CAD build for the part. Positions are in the model's coordinates, mm. A direction names the side the tool comes from. Coordinates: 2 decimals unless noted, no trailing zeros. Loops run counter-clockwise (first coordinate to the right, second up) from the corner with the lowest first, then second, coordinate; pieces in that order, holes last. Notation, with made-up numbers: (57, -10) -> (79, -10) arc R20 cw to (79, 19) -> close; hole circle Ø11 at (-31, 16). An arc over 180 degrees is marked (long way). Answer as CSV lines item,"result". Start each with the question number.
Autodesk Inventor part; units mm, degrees
ref_plane "YZ Plane" through (0, 0, 0) normal (1, 0, 0) x (0, 1, 0)
ref_plane "XZ Plane" through (0, 0, 0) normal (0, 1, 0) x (-1, 0, 0)
ref_plane "XY Plane" through (0, 0, 0) normal (0, 0, 1) x (1, 0, 0)
sketch "Sketch1" plane through (0, 0, 0) normal (0, 1, 0) x (-1, 0, 0)
  line L0 (-7.5, 35) -> (7.5, 35)
  line L1 (7.5, 35) -> (7.5, -35)
  line L2 (7.5, -35) -> (-7.5, -35)
  line L3 (-7.5, -35) -> (-7.5, 35)
  line L4 (-7.5, 35) -> (7.5, -35) construction
  line L5 (7.5, 35) -> (-7.5, -35) construction
  circle A0 centre (0, 17) radius 1.75
  circle A1 centre (0, -17) radius 1.75
  point P0 (0, 0)
  point P1 (0, -35)
  dimension "d0" = 15
  dimension "d1" = 70
  dimension "d13" = 18
  dimension "d14" = 18
  dimension "d16" = 3.5
extrude "Extrusion1" add sketch "Sketch1" along normal blind 3
sketch "Sketch2" plane through (-7.5, 0, 35) normal (0, 0, 1) x (1, 0, 0)
  line L0 (0, 0) -> (15, 0)
  line L1 (15, 0) -> (15, 3)
  line L2 (0, 3) -> (15, 3)
  line L3 (0, 0) -> (0, 3)
  line L4 (15, 3) -> (0, 3)
  line L5 (0, 3) -> (15, 3)
  line L6 (15, 3) -> (15, 18)
  line L7 (15, 18) -> (0, 18)
  line L8 (0, 18) -> (0, 3)
  circle A0 centre (7.5, 10.5) radius 1.75
  point P0 (7.5, 0)
  point P1 (7.5, 18)
  point P2 (0, 10.5)
  dimension "d15" = 3.5
extrude "Extrusion2" add sketch "Sketch2" against normal blind 3 contours L8 L7 L6 L2
sketch "Sketch3" plane through (7.5, 0, -35) normal (0, 0, -1) x (-1, 0, 0)
  line L0 (15, 18) -> (0, 18)
  line L1 (0, 18) -> (0, 3)
  line L2 (15, 3) -> (0, 3)
  line L3 (15, 3) -> (15, 18)
  circle A0 centre (7.5, 10.5) radius 1.75
  point P0 (7.5, 0)
extrude "Extrusion3" add sketch "Sketch3" against normal blind 3
sketch "Sketch4" plane through (7.5, 0, 35) normal (1, 0, 0) x (0, 0, -1)
  line L0 (0, 0) -> (70, 0)
  line L1 (70, 0) -> (70, 18)
  line L2 (70, 18) -> (67, 18)
  line L3 (67, 3) -> (67, 18)
  line L4 (3, 3) -> (67, 3)
  line L5 (3, 18) -> (3, 3)
  line L6 (0, 18) -> (3, 18)
  line L7 (0, 0) -> (0, 18)
  line L8 (3, 18) -> (18, 3)
  line L9 (67, 3) -> (67, 18)
  line L10 (67, 18) -> (52, 3)
  line L11 (67, 3) -> (3, 3)
  point P0 (35, 0)
  dimension "d8" = 45
extrude "Extrusion4" add sketch "Sketch4" against normal blind 2 contours L8 L4 L5 | L3 L4 L10
sketch "Sketch5" plane through (-7.5, 0, -35) normal (-1, 0, 0) x (0, 0, 1)
  line L0 (18, 3) -> (3, 3)
  line L1 (18, 3) -> (3, 18)
  line L2 (3, 3) -> (3, 18)
  line L3 (67, 3) -> (52, 3)
  line L4 (67, 18) -> (67, 3)
  line L5 (67, 18) -> (52, 3)
  point P0 (35, 0)
extrude "Extrusion5" add sketch "Sketch5" against normal blind 2
equation "\"d14\" = d13"
properties part number "Frame_Brace_Mount" material "ABS Plastic"
Item 1: Wall check: probe 1 along Z at (x, y) = (0, 0.7); probe 2 along Z at (x, y) = (-0.5, 5.75); probe 3 along Y at (x, z) = (0, 33.8). Give the ranges that are in metal, low to high.
Item 2: Which spindle directions (+Z, -Z, +X, -X, +Y, -Y) get a long thin tool onto all of the face, cutting with end or side? Do faces 1 (the face through (1.3, 12.3, -32)), 2 (the face through (7.5, 1, 0)), 3 (the face through (7, 11, 25)). Say none if no direction does.
Item 3: Two-plate mould, pull along Y, no slides. Class faces 4 (the face through (-7, 11, 25)), 5 (the face through (0.228, 1.479, 15.265)), 6 (the face through (0.228, 12.235, -33.521)), 7 (the face through (-0.228, 12.235, 33.521)): pulls with the +Y half, pulls with the -Y half, needs draft (parallel to the pull), parting line crosses it, or undercut.
Item 4: Saw through at B-B (y = 16). Write the cut outline in (x, z), plus the area to 3 significant figures.
Item 5: Saw through at A-A (x = 0). Write the cut outline in (y, z), plus the area to 3 significant figures.
Item 6: Saw through at C-C (z = 26). Write the cut outline in (x, y).
Item 7: Saw through at D-D (x = 4). Write the cut outline in (y, z), plus the area to 3 significant figures.
Geometry check:
1,probe 1,"-35 to -18.75, -15.25 to 15.25, 18.75 to 35"
1,probe 2,"-35 to -32, 32 to 35"
1,probe 3,"0 to 8.75, 12.25 to 18"
2,face 1,"+Y"
2,face 2,"+Z, -Z, +X, +Y, -Y"
2,face 3,"+X, -X, +Y"
3,face 4,"pulls with the +Y half"
3,face 5,"needs draft"
3,face 6,"undercut"
3,face 7,"undercut"
4,outline,"(-7.5, -35) -> (7.5, -35) -> (7.5, -30) -> (5.5, -30) -> (5.5, -32) -> (-5.5, -32) -> (-5.5, -30) -> (-7.5, -30) -> close; (-7.5, 30) -> (-5.5, 30) -> (-5.5, 32) -> (5.5, 32) -> (5.5, 30) -> (7.5, 30) -> (7.5, 35) -> (-7.5, 35) -> close"
4,area,"106 mm2"
5,outline,"(0, -35) -> (8.75, -35) -> (8.75, -32) -> (3, -32) -> (3, -18.75) -> (0, -18.75) -> close; (0, -15.25) -> (3, -15.25) -> (3, 15.25) -> (0, 15.25) -> close; (0, 18.75) -> (3, 18.75) -> (3, 32) -> (8.75, 32) -> (8.75, 35) -> (0, 35) -> close; (12.25, -35) -> (18, -35) -> (18, -32) -> (12.25, -32) -> close; (12.25, 32) -> (18, 32) -> (18, 35) -> (12.25, 35) -> close"
5,area,"258 mm2"
6,outline,"(-7.5, 0) -> (7.5, 0) -> (7.5, 12) -> (5.5, 12) -> (5.5, 3) -> (-5.5, 3) -> (-5.5, 12) -> (-7.5, 12) -> close"
7,outline,"(0, -35) -> (18, -35) -> (18, -32) -> (3, -32) -> (3, 32) -> (18, 32) -> (18, 35) -> (0, 35) -> close"
7,area,"300 mm2"
